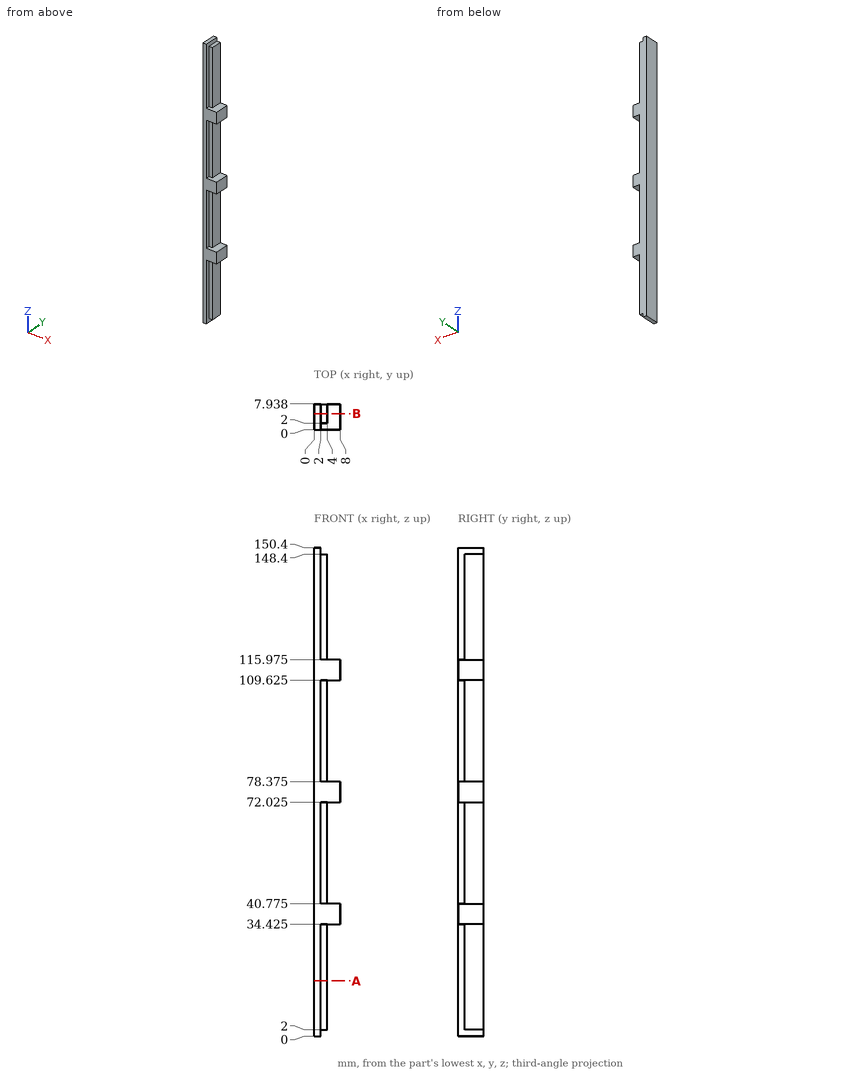
Input: dimensioned drawing with shaded views. Units: mm. Origin: part minimum x, y, z. Coordinates: 2 decimals unless noted, no trailing zeros. Loops run counter-clockwise (first coordinate to the right, second up) from the corner with the lowest first, then second, coordinate; pieces in that order, holes last. Notation, with made-up numbers: M 6.5,10.25 L 36.5,10.25 A21 cw 36.5,45.25 Z; hole C 21.25,-26 d4. An arc over 180 degrees is marked long. Use a Markdown table: item, result. Add a question column.
Q1. Section query B-B, the plane y = 5. Return loops of the section in (x, z) (1 decimal).
Q2. Section query A-A, the plane z = 17. Return loops of the section in (x, y).
Q3. First-contact query: pin 1 (1.6 mm diameter, centred on x = 3, y = 6, fed in from +Z); pin 2 (1 mm diameter, centred on x = 3, z = 134.5, fed in from -Y); pin 3 (2 mm diameter, centred on y = 4, z = 33, fed in from +X). Flat tips, straight axial feed; report the tip coordinate or a pass-through.
Q4. Material intervals for L1, parallel to Z at x = 4.25, y = 3.75 (1 decimal); L2, parallel to X at y = 6.75, z = 138; L3, parallel to Y at x = 3.75, z = 141.5, sorted ascending.
Result:
| question | item | result |
|---|---|---|
| 1 | outline | M 0,0 L 2,0 L 2,2 L 4,2 L 4,34.4 L 8,34.4 L 8,40.8 L 4,40.8 L 4,72 L 8,72 L 8,78.4 L 4,78.4 L 4,109.6 L 8,109.6 L 8,116 L 4,116 L 4,148.4 L 2,148.4 L 2,150.4 L 0,150.4 Z |
| 2 | outline | M 0,0 L 2,0 L 2,2 L 4,2 L 4,7.94 L 0,7.94 Z |
| 3 | pin 1 | stops at z = 148.4 |
| 3 | pin 2 | stops at y = 2 |
| 3 | pin 3 | stops at x = 4 |
| 4 | L1 | z = 34.4 to 40.8, 72 to 78.4, 109.6 to 116 |
| 4 | L2 | x = 0 to 4 |
| 4 | L3 | y = 2 to 7.94 |
